CAD build for the part. Positions are in the model's coordinates, mm. Round coordinates to 2 decimals unless told otherwise and drop trailing zeros. Loops run counter-clockwise (first coordinate to the right, second up) from the corner with the lowest first, then second, coordinate; pieces in that order, holes last. Notation, with made-up numbers: M 51.5,65 L 59.5,65 A11 ccw 59.5,83 Z; hole C 57.25,-6 d11. An arc over 180 degrees is marked long. Use one line per item in the form item = value.
from build123d import *

# Parameters (mm, degrees)
SKETCH1_R               = 3.175
BOSS_EXTRUDE1_DEPTH     = 50.8
CUT_EXTRUDE1_DEPTH      = 12.192
CUT_EXTRUDE1_DEPTH_BACK = 11.176
SKETCH2_R               = 1.5875
CUT_EXTRUDE2_DEPTH      = 11.176
CUT_EXTRUDE2_DEPTH_BACK = 11.176
SKETCH3_R               = 1.5875


with BuildPart() as part:
    # Sketch1 → Boss-Extrude1 (new body)
    with BuildSketch(Plane(origin=(0, 0, 0), x_dir=(1, 0, 0), z_dir=(0, 1, 0))):
        with Locations(Location((0, 0, 0), (0, 0, 270))):
            Circle(SKETCH1_R)
    extrude(amount=BOSS_EXTRUDE1_DEPTH)

    # Sketch2 → Cut-Extrude1 (cut, two sides: drawn at the far end of the back side and taken through both)
    with BuildSketch(Plane.XY.offset(-CUT_EXTRUDE1_DEPTH_BACK)):
        with Locations(Location((0, 43.18, 0), (0, 0, 89.99999999))):
            Circle(SKETCH2_R)
    extrude(amount=CUT_EXTRUDE1_DEPTH + CUT_EXTRUDE1_DEPTH_BACK, mode=Mode.SUBTRACT)

    # Sketch3 → Cut-Extrude2 (cut, two sides: drawn at the far end of the back side and taken through both)
    with BuildSketch(Plane.XY.offset(-CUT_EXTRUDE2_DEPTH_BACK)):
        with Locations(Location((0, 7.62, 0), (0, 0, 89.99999999))):
            Circle(SKETCH3_R)
    extrude(amount=CUT_EXTRUDE2_DEPTH + CUT_EXTRUDE2_DEPTH_BACK, mode=Mode.SUBTRACT)


solid = part.part
1. Cut at D-D on z = 2.5. Write the cut outline in (x, y) (1 decimal).
Completed:
outline = M -2,0 L 2,0 L 2,50.8 L -2,50.8 Z; hole C 0,7.6 d3.2; hole C 0,43.2 d3.2
2. Drop flat-ended pins along their axis: P1, Ø1.5, axis at x = 0.5, y = 42, coming from the -Z side (3 decimals); P2, Ø1.9, axis at x = 0, y = 7.62, coming from the -Z side; P3, Ø1, axis at x = 2, y = 30, coming from the -Z side. Give the stop position or say it passes through.
Completed:
P1 = -3.175
P2 = through
P3 = -2.8
3. Cut at B-B on y = 14. Write the cut outline in (x, z) (3 decimals).
Completed:
outline = C 0,0 d6.35
4. Pull direction Y, two halves, no side cores. Call faces 1 (the face through (0, 0, 0)), 2 (the face through (-1.34, 8.47, -0.05)), 3 (the face through (0, 50.8, 0)), 4 (the face through (-1.34, 44.03, -0.05)): +Y half, -Y half, draft (parallel to the pull), parting line (faces both ways), or undercut.
Completed:
face_1 = -Y half
face_2 = undercut
face_3 = +Y half
face_4 = undercut
5. Cut at A-A on z = 0. Write the cut outline in (x, y) (1 decimal), and give its area (3 significant figures).
Completed:
outline = M -3.2,0 L 3.2,0 L 3.2,50.8 L -3.2,50.8 Z; hole C 0,7.6 d3.2; hole C 0,43.2 d3.2
area = 307 mm2
6. Probe line 1 along Y through (x, z) = (0.5, -0.5); line 2 along Y through (x, z) = (-1, -0.5); line 3 along Z through (x, y) = (0.25, 23). List the from-to ranges inside material, lowest first. Write a range as from..to.
Completed:
line_1 = 0..6.11, 9.13..41.67, 44.69..50.8
line_2 = 0..6.39, 8.85..41.95, 44.41..50.8
line_3 = -3.17..3.17
